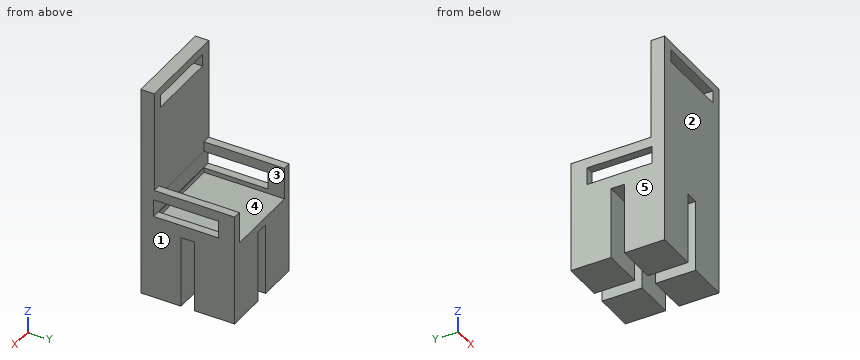
from build123d import *

# Parameters (mm, degrees)
F0_W      = 15
F0_H      = 15
F1_DEPTH  = 30
F3_W      = 35
F3_H      = 35
F4_DEPTH  = 3
F5_W      = 35
F5_H      = 5
F6_DEPTH  = 50
F7_W      = 27
F7_H      = 4.6730685326
F8_DEPTH  = 25
F9_W      = 3
F9_H      = 30
F10_DEPTH = 12
F12_W     = 24.1443798877
F12_H     = 6.5082572401
F11_W     = 23.8036615774
F11_H     = 4.3690986931
F13_DEPTH = 349


with BuildPart() as f1:
    # F0 (on Top) → F1 (new body)
    with BuildSketch(Plane.XY):
        with Locations((7.5, 7.5)):
            Rectangle(F0_W, F0_H)
    extrude(amount=F1_DEPTH)



with BuildPart() as f1b:
    # F0 (on Top) → F1, piece 2 (new body)
    with BuildSketch(Plane.XY):
        with Locations((7.5, 27.5)):
            Rectangle(F0_W, F0_H)
    extrude(amount=F1_DEPTH)


with BuildPart() as f1c:
    # F0 (on Top) → F1, piece 3 (new body)
    with BuildSketch(Plane.XY):
        with Locations((27.5, 27.5)):
            Rectangle(F0_W, F0_H)
    extrude(amount=F1_DEPTH)


with BuildPart() as f1d:
    # F0 (on Top) → F1, piece 4 (new body)
    with BuildSketch(Plane.XY):
        with Locations((27.5, 7.5)):
            Rectangle(F0_W, F0_H)
    extrude(amount=F1_DEPTH)


with BuildPart() as f1_1:
    add(f1.part)

    add(f1b.part)  # F4 merges F1b

    add(f1c.part)  # F4 merges F1c

    add(f1d.part)  # F4 merges F1d
    # F3 (on face) → F4 (join)
    with BuildSketch(Plane.XY.offset(30)):
        with Locations((17.5, 17.5)):
            Rectangle(F3_W, F3_H)
    extrude(amount=-F4_DEPTH)

    # F5 (on face) → F6 (join)
    with BuildSketch(Plane.XY.offset(30)):
        with Locations((17.5, 2.5)):
            Rectangle(F5_W, F5_H)
    extrude(amount=F6_DEPTH)

    # F7 (on face) → F8 (cut)
    with BuildSketch(Plane.XZ):
        with Locations((17.5, 74.6634657337)):
            Rectangle(F7_W, F7_H)
    extrude(amount=-F8_DEPTH, mode=Mode.SUBTRACT)

    # F9 (on face) → F10 (join)
    with BuildSketch(Plane.XY.offset(30)):
        with Locations((33.5, 20)):
            Rectangle(F9_W, F9_H)
        with Locations((1.5, 20)):
            Rectangle(F9_W, F9_H)
    extrude(amount=F10_DEPTH)

    # F12 (on face) + F11 (on face) → F13 (cut)
    with BuildSketch(Plane(origin=(0, 0, 0), x_dir=(0, -1, 0), z_dir=(-1, 0, 0))):
        with Locations((-16.8588969391, 34.9941607565)):
            Rectangle(F12_W, F12_H)
    with BuildSketch(Plane.YZ.offset(35)):
        with Locations((19.5460454561, 34.8994340748)):
            Rectangle(F11_W, F11_H)
    extrude(amount=-F13_DEPTH, dir=(-1, 0, 0), mode=Mode.SUBTRACT)


solid = f1_1.part
The model under review builds one solid part; all positions refer to its coordinate system, in mm. Face numbers are marked on the shaded views. A direction names the side the tool comes from. Give positions to 0.01 mm unless a question says otherwise; leave off trailing zeros. Loops run counter-clockwise (first coordinate to the right, second up) from the corner with the lowest first, then second, coordinate; pieces in that order, holes last. Notation, with made-up numbers: (81, -31) -> (140, -31) arc R14 ccw to (140, -10) -> close; hole circle Ø9 at (70, 37). An arc over 180 degrees is marked (long way). Answer as a JSON object with one key per item and string values. Group by question number.
Q1. Take a section at A-A (z = 36). Write out the cut boundary in (x, y), plus the area to 3 significant figures.
Q2. Take a section at D-D (y = 16). Write out the cut boundary in (x, z).
Q3. Take a section at C-C (z = 25). Write out the cut boundary in (x, y), plus the area to 3 significant figures.
Q4. Wall thickness on line 1 along Y through (x, z) = (27, 6.5); line 2 along Z through (x, y) = (14.5, 3): over which ranges is each line inside the solid? List them lowest first.
Q5. Insertion check: pin 1 (1.9 mm diameter, centred on x = 21.5, z = 31, fed in from +Y); pin 2 (0.9 mm diameter, centred on x = 1, y = 13.5, fed in from +Z). Each pin has a flat end and moves straight along its axis. Give the tip position at first contact, or say it passes through.
Q6. Tool access review of the marked faces 4 and 5: name each direction out of +Z, -Z, +X, -X, +Y, -Y from which nothing blocks a thin tool from reaching the whole face with its end or side.
Q7. Draft analysis for pull direction X (two halves, no side actions). For the marked faces 1, 2 and 3, state which applies: pulls with the +X half, pulls with the -X half, needs draft (parallel to the pull), parting line crosses it, or undercut.
Q8. Take a section at B-B (x = 8). Write out the cut boundary in (y, z), plus the area to 3 significant figures.
Answer below:
{
 "1": {"outline": "(0, 0) -> (35, 0) -> (35, 4.79) -> (0, 4.79) -> close; (0, 28.93) -> (3, 28.93) -> (3, 35) -> (0, 35) -> close; (32, 28.93) -> (35, 28.93) -> (35, 35) -> (32, 35) -> close", "area": "204 mm2"},
 "2": {"outline": "(0, 27) -> (35, 27) -> (35, 31.74) -> (32, 31.74) -> (32, 30) -> (3, 30) -> (3, 31.74) -> (0, 31.74) -> close; (0, 38.25) -> (3, 38.25) -> (3, 42) -> (0, 42) -> close; (32, 38.25) -> (35, 38.25) -> (35, 42) -> (32, 42) -> close"},
 "3": {"outline": "(0, 0) -> (15, 0) -> (15, 15) -> (0, 15) -> close; (0, 20) -> (15, 20) -> (15, 35) -> (0, 35) -> close; (20, 0) -> (35, 0) -> (35, 15) -> (20, 15) -> close; (20, 20) -> (35, 20) -> (35, 35) -> (20, 35) -> close", "area": "900 mm2"},
 "4": {"line 1": "y = 0 to 15, 20 to 35", "line 2": "z = 0 to 72.33, 77 to 80"},
 "5": {"pin 1": "stops at y = 5", "pin 2": "stops at z = 42"},
 "6": {"face 4": "+Z, +Y", "face 5": "+Z, -Z, -X, +Y, -Y"},
 "7": {"face 1": "pulls with the +X half", "face 2": "needs draft", "face 3": "undercut"},
 "8": {"outline": "(0, 0) -> (15, 0) -> (15, 27) -> (20, 27) -> (20, 0) -> (35, 0) -> (35, 30) -> (5, 30) -> (5, 31.74) -> (4.79, 31.74) -> (4.79, 38.25) -> (5, 38.25) -> (5, 72.33) -> (0, 72.33) -> close; (0, 77) -> (5, 77) -> (5, 80) -> (0, 80) -> close", "area": "1,140 mm2"}
}
